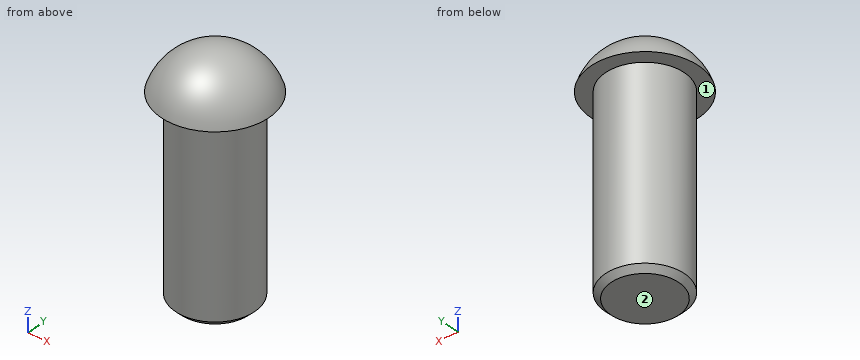
```python
from build123d import *

# Parameters (mm, degrees)
ESQUISSE1_R          = 3.5
BASE_EXTRUSION_DEPTH = 17
CHANFREIN1_SIZE      = 0.5


with BuildPart() as part:
    # Esquisse1 → Base-Extrusion (new body)
    with BuildSketch(Plane.XY):
        Circle(ESQUISSE1_R)
    extrude(amount=-BASE_EXTRUSION_DEPTH)

    # Esquisse3 → Boss.-Révol.1 (revolve)
    with BuildSketch(Plane(origin=(0, 0, 0), x_dir=(0, 0, -1), z_dir=(1, 0, 0))):
        with BuildLine():
            Line((0, 0), (0, 4.769696007))
            ThreePointArc((0, 4.769696007), (-2.531128874, 2.958039892), (-3.5, 0))
            Line((-3.5, 0), (0, 0))
        make_face()
    revolve(axis=Axis((0, 0, 0), (0, 0, -1)))

    # Chanfrein1
    chanfrein1_edges = [part.edges().sort_by_distance(p)[0] for p in [
        (-3.5, 0, -17),
    ]]
    chamfer(chanfrein1_edges, length=CHANFREIN1_SIZE)


solid = part.part
```
Input: part model. Units: mm. Frame: model coordinates. Face numbers are marked on the shaded views. A direction names the side the tool comes from. Give positions to 0.01 mm unless a question says otherwise; leave off trailing zeros. Order: outer loops, then holes, each group sorted by start corner. A loop starts at its lowest first (then second) coordinate and runs counter-clockwise, first axis right, second up. Notation, with made-up numbers: M 67,33 L 110,33 A19 cw 110,54 Z; hole C -32,-33 d7. An arc over 180 degrees is marked long. Return JSON: item names as keys, results as strings.
Item 1: Access query for the marked faces 1 and 2. Directions: +Z, -Z, +X, -X, +Y, -Y. A direction counts if a zero-diameter tool reaches every point of the face in a straight line with its end or side. Return the directions, or none.
Solutions:
{"face 1": "-Z", "face 2": "-Z, +X, -X, +Y, -Y"}
Item 2: Cut plane D-D (z = 0.5). Return loops of the section in (x, y).
Solutions:
{"outline": "C 0,0 d9.17"}
Item 3: Cut plane C-C (z = -14). Return loops of the section in (x, y), then the cut area to 3 significant figures.
Solutions:
{"outline": "C 0,0 d7", "area": "38.5 mm^2"}
Item 4: Ray query, probe 1 along X at (y, z) = (-1.75, 2); probe 2 along Z at (x, y) = (-2.5, -0.5); probe 3 along X at (y, z) = (-2.25, -8.25). Return the intervals inside material, ascending.
Solutions:
{"probe 1": "-3.11 to 3.11", "probe 2": "-17 to 2.8", "probe 3": "-2.68 to 2.68"}
Item 5: Cut plane A-A (y = 0). Return loops of the section in (x, z).
Solutions:
{"outline": "M -4.77,0 L -3.5,0 L -3.5,-16.5 L -3,-17 L 3,-17 L 3.5,-16.5 L 3.5,0 L 4.77,0 A5 ccw Z"}
Item 6: First-contact query: P1, Ø3, axis at x = 3.5, z = -3.5, coming from the +Y side; P2, Ø1.5, axis at y = -1.5, z = -0.5, coming from the -X side; P3, Ø1, axis at x = -1.5, z = -12.5, coming from the +Y side. Flat tips, straight axial feed; report the tip coordinate or a pass-through.
Solutions:
{"P1": "y = 2.87", "P2": "x = -4.68", "P3": "y = 3.35"}
